Check sheet for the drawn part. Datum: minimum x, y, z corner. Units: mm. Give positions to 0.01 mm unless a question says otherwise; leave off trailing zeros. Write each loop counter-clockwise with the first axis right and the second up, starting at its lowest first coordinate (ties: lowest second). Pieces come first, ordered by that corner, then holes. Notation, with made-up numbers: M 68.25,54.5 L 90.25,54.5 A21 cw 90.25,62.5 Z; hole C 69,33.25 d10. An arc over 180 degrees is marked long. Use CSV: the item, a comma, the result in double quotes. Start each with the question number.
1. Scan lines: line 1 (Z direction, x = 10, y = 6.5); line 2 (Y direction, x = 8.75, z = 6). Record each from-to range of solid material in increasing order.
2. Cross-section at A-A, the plane y = 7.5. Enter the section's corners in (x, z), and give its area (3 significant figures).
3. Cross-section at B-B, the plane x = 6.25. Enter the section's corners in (y, z).
4. Cross-section at C-C, the plane z = 2.5. Enter the section's corners in (x, y).
5. Mould release check, pull along Z, two halves, no side actions. Record for the marked faces 1, 2, 3 and 4: +Z half, -Z half, draft (parallel to the pull), parting line (faces both ways), or undercut.
6. Depth check by flat-ended pin: P1, Ø1, axis at x = 16.5, z = 3, coming from the -Y side. Enter the tip coordinate at first touch or a pass-through.
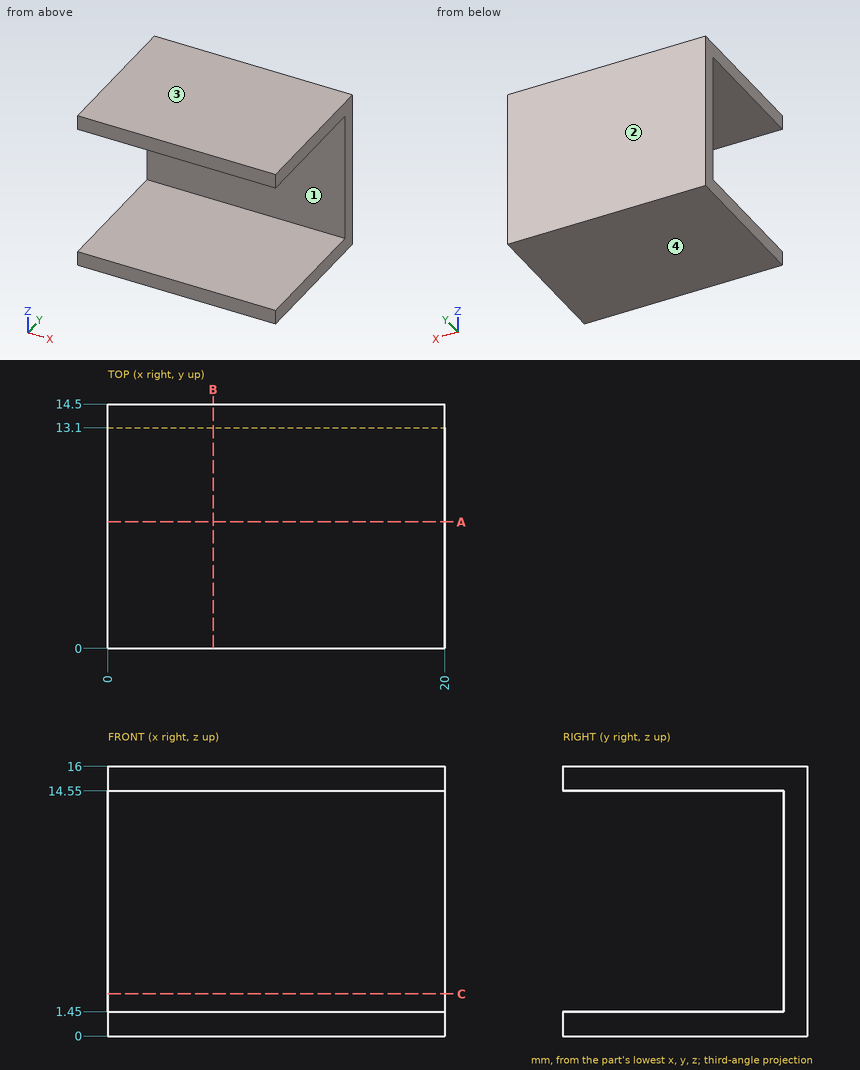
Worked answers:
1,line 1,"z = 0 to 1.45, 14.55 to 16"
1,line 2,"y = 13.1 to 14.5"
2,outline,"M 0,0 L 20,0 L 20,1.45 L 0,1.45 Z; M 0,14.55 L 20,14.55 L 20,16 L 0,16 Z"
2,area,"58.0 mm^2"
3,outline,"M 0,0 L 14.5,0 L 14.5,16 L 0,16 L 0,14.55 L 13.1,14.55 L 13.1,1.45 L 0,1.45 Z"
4,outline,"M 0,13.1 L 20,13.1 L 20,14.5 L 0,14.5 Z"
5,face 1,"undercut"
5,face 2,"draft"
5,face 3,"+Z half"
5,face 4,"-Z half"
6,P1,"stops at y = 13.1"
